from build123d import *

# Parameters (mm, degrees)
SKETCH_1_R         = 60
SKETCH_1_R_2       = 1.55
SKETCH_1_R_3       = 2.1
SKETCH_1_R_4       = 6
EXTRUDE_1_DEPTH    = 3
SKETCH1_R          = 2.15
CUT_EXTRUDE1_DEPTH = 10


with BuildPart() as part:
    # 草图1 → 凸台-拉伸1 (new body)
    with BuildSketch(Plane.XY):
        Circle(SKETCH_1_R)
        with Locations((0, 54.5)):
            Circle(SKETCH_1_R_2, mode=Mode.SUBTRACT)
        with Locations((-54.5, 0)):
            Circle(SKETCH_1_R_2, mode=Mode.SUBTRACT)
        with Locations((0, -54.5)):
            Circle(SKETCH_1_R_2, mode=Mode.SUBTRACT)
        with Locations((54.5, 0)):
            Circle(SKETCH_1_R_2, mode=Mode.SUBTRACT)
        with Locations((14.142135624, 14.142135624)):
            Circle(SKETCH_1_R_3, mode=Mode.SUBTRACT)
        with Locations((5.176380902, -19.318516526)):
            Circle(SKETCH_1_R_3, mode=Mode.SUBTRACT)
        with Locations((-19.318516526, 5.176380902)):
            Circle(SKETCH_1_R_3, mode=Mode.SUBTRACT)
        Circle(SKETCH_1_R_4, mode=Mode.SUBTRACT)
        with BuildLine():
            Line((3.923217687, -28.453617749), (6.022703538, -43.680396542))
            ThreePointArc((6.022703538, -43.680396542), (8.67451724, -47.877141015), (13.579927123, -48.639855873))
            ThreePointArc((13.579927123, -48.639855873), (35.70889245, -35.70889245), (48.639855873, -13.579927123))
            ThreePointArc((48.639855873, -13.579927123), (47.877141015, -8.67451724), (43.680396542, -6.022703538))
            Line((43.680396542, -6.022703538), (28.453617749, -3.923217687))
            ThreePointArc((28.453617749, -3.923217687), (25.717860997, -4.538114468), (24.057984584, -6.7980422))
            ThreePointArc((24.057984584, -6.7980422), (17.67766953, -17.67766953), (6.7980422, -24.057984584))
            ThreePointArc((6.7980422, -24.057984584), (4.538114468, -25.717860997), (3.923217687, -28.453617749))
        make_face(mode=Mode.SUBTRACT)
        with BuildLine():
            Line((28.453617749, 3.923217687), (43.680396542, 6.022703538))
            ThreePointArc((43.680396542, 6.022703538), (47.877141015, 8.67451724), (48.639855873, 13.579927123))
            ThreePointArc((48.639855873, 13.579927123), (35.70889245, 35.70889245), (13.579927123, 48.639855873))
            ThreePointArc((13.579927123, 48.639855873), (8.67451724, 47.877141015), (6.022703538, 43.680396542))
            Line((6.022703538, 43.680396542), (3.923217687, 28.453617749))
            ThreePointArc((3.923217687, 28.453617749), (4.538114468, 25.717860997), (6.7980422, 24.057984584))
            ThreePointArc((6.7980422, 24.057984584), (17.67766953, 17.67766953), (24.057984584, 6.7980422))
            ThreePointArc((24.057984584, 6.7980422), (25.717860997, 4.538114468), (28.453617749, 3.923217687))
        make_face(mode=Mode.SUBTRACT)
        with BuildLine():
            Line((-28.453617749, -3.923217687), (-43.680396542, -6.022703538))
            ThreePointArc((-43.680396542, -6.022703538), (-47.877141015, -8.67451724), (-48.639855873, -13.579927123))
            ThreePointArc((-48.639855873, -13.579927123), (-35.70889245, -35.70889245), (-13.579927123, -48.639855873))
            ThreePointArc((-13.579927123, -48.639855873), (-8.67451724, -47.877141015), (-6.022703538, -43.680396542))
            Line((-6.022703538, -43.680396542), (-3.923217687, -28.453617749))
            ThreePointArc((-3.923217687, -28.453617749), (-4.538114468, -25.717860997), (-6.7980422, -24.057984584))
            ThreePointArc((-6.7980422, -24.057984584), (-17.67766953, -17.67766953), (-24.057984584, -6.7980422))
            ThreePointArc((-24.057984584, -6.7980422), (-25.717860997, -4.538114468), (-28.453617749, -3.923217687))
        make_face(mode=Mode.SUBTRACT)
        with BuildLine():
            Line((-3.923217687, 28.453617749), (-6.022703538, 43.680396542))
            ThreePointArc((-6.022703538, 43.680396542), (-8.67451724, 47.877141015), (-13.579927123, 48.639855873))
            ThreePointArc((-13.579927123, 48.639855873), (-35.70889245, 35.70889245), (-48.639855873, 13.579927123))
            ThreePointArc((-48.639855873, 13.579927123), (-47.877141015, 8.67451724), (-43.680396542, 6.022703538))
            Line((-43.680396542, 6.022703538), (-28.453617749, 3.923217687))
            ThreePointArc((-28.453617749, 3.923217687), (-25.717860997, 4.538114468), (-24.057984584, 6.7980422))
            ThreePointArc((-24.057984584, 6.7980422), (-17.67766953, 17.67766953), (-6.7980422, 24.057984584))
            ThreePointArc((-6.7980422, 24.057984584), (-4.538114468, 25.717860997), (-3.923217687, 28.453617749))
        make_face(mode=Mode.SUBTRACT)
    extrude(amount=EXTRUDE_1_DEPTH)

    # Sketch1 → Cut-Extrude1 (cut)
    with BuildSketch(Plane.XY.offset(3)):
        with Locations((50.167514513, -21.294846503)):
            Circle(SKETCH1_R)
        with Locations((21.294846503, -50.167514513)):
            Circle(SKETCH1_R)
    extrude(amount=-CUT_EXTRUDE1_DEPTH, mode=Mode.SUBTRACT)


solid = part.part
Input: part model. Units: mm. Frame: model coordinates. Coordinates: 2 decimals unless noted, no trailing zeros. Order: outer loops, then holes, each group sorted by start corner. A loop starts at its lowest first (then second) coordinate and runs counter-clockwise, first axis right, second up.
1. Ray query, line 1 along Y through (x, z) = (0, 2.35); line 2 along Y through (x, z) = (14.5, 1.25); line 3 along Y through (x, z) = (34.5, 2.15). Return the intervals inside material, ascending.
Checked values:
line 1: y = -60 to -56.05, -52.95 to -6, 6 to 52.95, 56.05 to 60
line 2: y = -58.22 to -48.37, -20.37 to 12.07, 16.21 to 20.37, 48.37 to 58.22
line 3: y = -49.09 to -36.88, -4.76 to 4.76, 36.88 to 49.09
2. Draft query along Y for faces 1 (the flat face through (36.174, -4.988, 1.479)), 2 (the flat face through (-1, -12, 0)). Return one class per face: +Y half, -Y half, draft (parallel to the pull), parting line (faces both ways), or undercut.
Checked values:
face 1: undercut
face 2: draft
3. Contact query for a flat-ended pin moving along its axis: P1, Ø7, axis at x = 50.17, y = -21.29, coming from the +Z side. Output: stop coordinate, or through.
Checked values:
P1: stops at z = 3
4. Cut plane A-A, the plane y = 0. Return loops of the section in (x, z).
Checked values:
outline: (-60, 0) - (-56.05, 0) - (-56.05, 3) - (-60, 3) - close; (-52.95, 0) - (-6, 0) - (-6, 3) - (-52.95, 3) - close; (6, 0) - (52.95, 0) - (52.95, 3) - (6, 3) - close; (56.05, 0) - (60, 0) - (60, 3) - (56.05, 3) - close
5. Cut plane C-C, the plane x = 54.5. Return loops of the section in (y, z).
Checked values:
outline: (-25.09, 0) - (-1.55, 0) - (-1.55, 3) - (-25.09, 3) - close; (1.55, 0) - (25.09, 0) - (25.09, 3) - (1.55, 3) - close
